Can you work these out from the model? Positions are in its coordinate system, mm. Give positions to 0.01 mm unless a question says otherwise; leave off trailing zeros. Order: outer loops, then holes, each group sorted by start corner. A loop starts at its lowest first (then second) coordinate and runs counter-clockwise, first axis right, second up. Notation, with made-up numbers: (-35.5, -12.75) - (-30.5, -12.75) arc R20 ccw to (-30.5, 14.25) - close; hole circle Ø10 at (86, -38). An arc over 180 degrees is marked (long way). One line per question, with ' | ' between items.
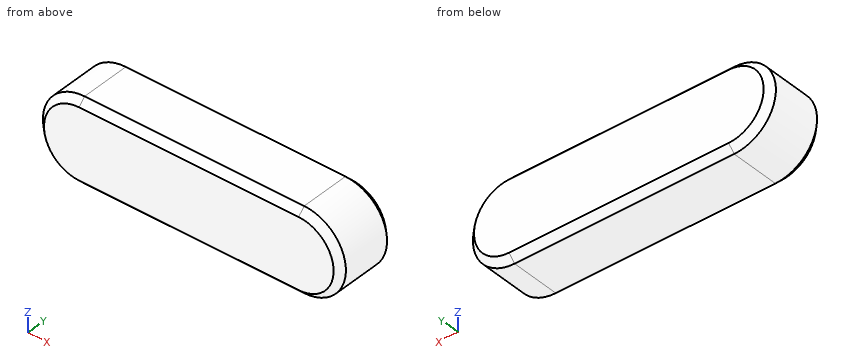
```python
from build123d import *

# Parameters (mm, degrees)
F0_W     = 66.7258
F0_H     = 12.6746
F1_DEPTH = 19.05
F2_SIZE  = 2.032
F3_SIZE  = 2.032


with BuildPart() as f1:
    # F0 (on Front) → F1 (new body)
    with BuildSketch(Plane.XZ):
        with BuildLine():
            ThreePointArc((0, 25.3492), (-12.6746, 12.6746), (0, 0))
            Line((0, 0), (0, 12.6746))
            Line((0, 12.6746), (0, 25.3492))
        make_face()
        with Locations((33.3629, 19.0119)):
            Rectangle(F0_W, F0_H)
        with Locations((33.3629, 6.3373)):
            Rectangle(F0_W, F0_H)
        with BuildLine():
            Line((66.7258, 12.6746), (66.7258, 0))
            ThreePointArc((66.7258, 0), (79.4004, 12.6746), (66.7258, 25.3492))
            Line((66.7258, 25.3492), (66.7258, 12.6746))
        make_face()
    extrude(amount=F1_DEPTH)

    # F2
    f2_edges = [f1.edges().sort_by_distance(p)[0] for p in [
        (-12.6746, 0, 12.6746),
        (33.3629, 0, 0),
        (79.4004, 0, 12.6746),
        (33.3629, 0, 25.3492),
    ]]
    chamfer(f2_edges, length=F2_SIZE)

    # F3
    f3_edges = [f1.edges().sort_by_distance(p)[0] for p in [
        (-12.6746, -19.05, 12.6746),
        (33.3629, -19.05, 0),
        (79.4004, -19.05, 12.6746),
        (33.3629, -19.05, 25.3492),
    ]]
    chamfer(f3_edges, length=F3_SIZE)


solid = f1.part
```
(1) Imagine slicing it at A-A (x = 22.5). List the corners of the cut face in (y, z) for me, and give its area (3 significant figures).
Answer below:
outline: (-19.05, 2.03) - (-17.02, 0) - (-2.03, 0) - (0, 2.03) - (0, 23.32) - (-2.03, 25.35) - (-17.02, 25.35) - (-19.05, 23.32) - close | area: 475 mm^2
(2) If I drill on line 1 (X direction, y = -4, z = 2.25); line 2 (X direction, y = -13.5, z = 3); line 3 (Y direction, x = 25.5, z = 23.75), over which ranges is the centre line in solid material (lowest first)?
Answer below:
line 1: -7.21 to 73.94 | line 2: -8.19 to 74.91 | line 3: -18.62 to -0.43
(3) Will these pins go through, and if not, where does the flat tip stop? pin 1 (5 mm diameter, centred on y = -13, z = 10.5, fed in from +X); pin 2 (1.5 mm diameter, centred on y = -13.5, z = 18, fed in from +X); pin 3 (1.5 mm diameter, centred on y = -11.5, z = 16, fed in from +X).
Answer below:
pin 1: x = 79.4 | pin 2: x = 78.55 | pin 3: x = 79.14
(4) Imagine slicing it at B-B (y = -5). List the corners of the cut face in (x, z) for me, and give its area (3 significant figures).
Answer below:
outline: (0, 0) - (66.73, 0) arc R12.67 ccw to (66.73, 25.35) - (0, 25.35) arc R12.67 ccw to start | area: 2,200 mm^2
